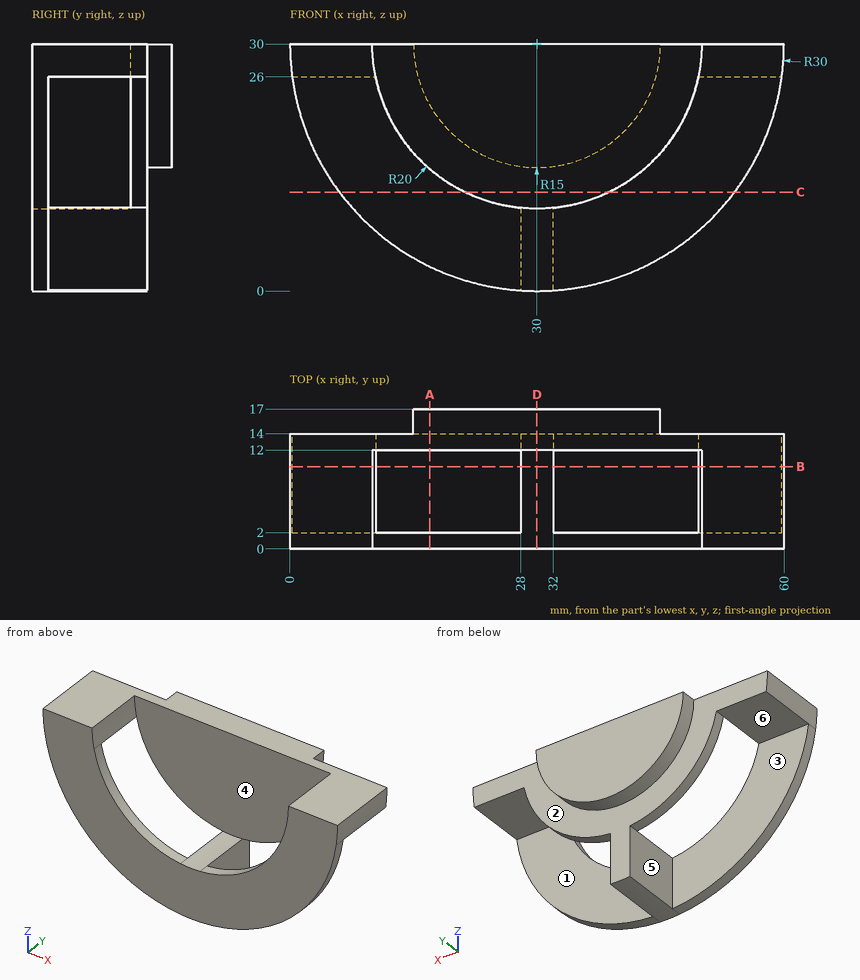
Can you work these out from the drawing? Everything is in mm from the part's minimum corner. A direction names the side the tool comes from. Give positions to 0.01 mm unless a question says otherwise; leave off trailing zeros. Order: outer loops, then holes, each group sorted by start corner. A loop starts at its lowest first (then second) coordinate and runs counter-clockwise, first axis right, second up.
Item 1: If we section it at D-D, the plane x = 30: Write out the boundary of the cut face in (y, z).
Item 2: If we section it at A-A, the plane x = 17: Write out the boundary of the cut face in (y, z), plus the area to 3 significant figures.
Item 3: If we section it at C-C, the plane z = 12: Write out the boundary of the cut face in (x, y).
Item 4: I need wall thicknesses on line 1 (Z direction, x = 30, y = 10.25); line 2 (X direction, y = 12, z = 8); line 3 (Y direction, x = 51, z = 13). Which ranges of each line are inside material? Lowest first, please.
Item 5: For the marked faces 1, 2 and 3, which set-ups out of +Z, -Z, +X, -X, +Y, -Y let a thin tool reach every point of the face, with its end or its side?
Item 6: If we mould it in two halves opening along X, with no side actions, what happens to the marked faces 4, 5 and 6? For each: pulls with the +X half, pulls with the -X half, needs draft (parallel to the pull), parting line crosses it, or undercut.
Item 7: I'm going to push flat-ended pins straight in: pin 1 (1.5 mm diameter, centred on x = 24.5, y = 14.5, fed in from -Z); pin 2 (5 mm diameter, centred on x = 54.5, y = 9.5, fed in from -Z); pin 3 (10 mm diameter, centred on x = 36, z = 16.5, fed in from -Y); pin 4 (1.5 mm diameter, centred on x = 13, z = 12.5, fed in from -Y). Where does each tip first touch, or does it pass through?
Item 8: If we section it at B-B, the plane y = 10: Write out the boundary of the cut face in (x, z).
Values:
1. outline: (0, 0) - (14, 0) - (14, 15) - (17, 15) - (17, 30) - (12, 30) - (12, 10) - (0, 10) - close
2. outline: (0, 2.96) - (2, 2.96) - (2, 14.8) - (0, 14.8) - close; (12, 14.8) - (14, 14.8) - (14, 22.52) - (17, 22.52) - (17, 30) - (12, 30) - close
2. area: 76.5 mm2
3. outline: (6, 0) - (21.28, 0) - (21.28, 2) - (6, 2) - close; (21.28, 12) - (38.72, 12) - (38.72, 14) - (21.28, 14) - close; (38.72, 0) - (54, 0) - (54, 2) - (38.72, 2) - close
4. line 1: z = 0 to 10
4. line 2: x = 28 to 32
4. line 3: y = 0 to 2
5. face 1: -Z, +X, +Y
5. face 2: -Z, +Y
5. face 3: -Z, -X, +Y
6. face 4: undercut
6. face 5: pulls with the -X half
6. face 6: needs draft
7. pin 1: stops at z = 10.62
7. pin 2: stops at z = 26
7. pin 3: stops at y = 12
7. pin 4: stops at y = 0
8. outline: (0, 30) arc R30 ccw to (0.27, 26) - (10.4, 26) arc R20 cw to (10, 30) - close; (28, 0.07) arc R30 ccw to (32, 0.07) - (32, 10.1) arc R20 cw to (28, 10.1) - close; (49.6, 26) - (59.73, 26) arc R30 ccw to (60, 30) - (50, 30) arc R20 cw to start
